Source: three-view drawing plus pictorial views. Frame: mm from the lowest corner of the part. Give positions to 0.01 mm unless a question says otherwise; leave off trailing zeros. Loops run counter-clockwise (first coordinate to the right, second up) from the corner with the lowest first, then second, coordinate; pieces in that order, holes last. Notation, with made-up numbers: (-1.75, 62) - (50.25, 62) arc R32 ccw to (50.25, 98) - close; hole circle Ø5 at (28, 81.5). An arc over 180 degrees is marked (long way). Answer as a JSON object with one key per item and string values.
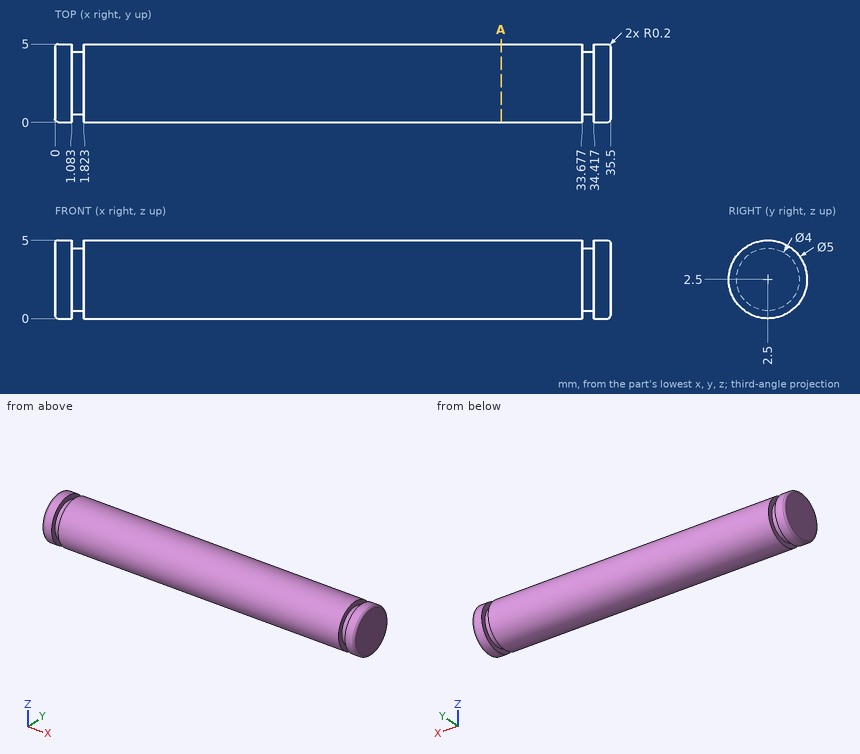
Item 1: Material intervals for line 1 (Z direction, x = 31, y = 2.6); line 2 (Y direction, x = 23, z = 1); line 3 (Y direction, x = 27, z = 4.5), sorted ascending. Write a range as [from, to].
Geometry check:
{"line 1": "z = [0, 5]", "line 2": "y = [0.5, 4.5]", "line 3": "y = [1, 4]"}
Item 2: Contact query for a flat-ended pin moving along its axis: P1, Ø1, axis at x = 31.5, y = 4, coming from the -Z side. Output: stop coordinate, or through.
Geometry check:
{"P1": "stops at z = 0.21"}
Item 3: Cut plane A-A (x = 28.5). Return loops of the section in (y, z), then the cut area to 3 significant figures.
Geometry check:
{"outline": "circle Ø5 at (2.5, 2.5)", "area": "19.6 mm2"}
